```python
from build123d import *

# Parameters (mm, degrees)
F0_W     = 1.5
F0_H     = 0.7
F0_R     = 2.25
F0_H_2   = 8.6
F0_W_2   = 2.8
F1_DEPTH = 5
F2_DEPTH = 3
F3_DEPTH = 2
F4_R     = 0.74999
F5_R     = 2


# Not quite as in the source:
# - a fillet or chamfer is up to 0.001 mm smaller than in the source, because OpenCascade refuses the exact size


with BuildPart() as f1:
    # F0 (on Top) → F1 (new body)
    with BuildSketch(Plane.XY):
        Polygon((-18.8879279066, 5), (-22.8879279066, 5), (-22.8879279066, 2), (-18.8879279066, 2.46), align=None)
        Polygon((-17.3879279066, 5), (-18.8879279066, 5), (-18.8879279066, 2.46), (-17.3879279066, 2.6325), align=None)
        Polygon((-18.8879279066, 2.46), (-22.8879279066, 2), (-22.8879279066, -2), (-18.8879279066, -2.46), align=None)
        Polygon((-12.9879279066, 5), (-17.3879279066, 5), (-17.3879279066, 2.6325), (-12.9879279066, 3.1385), align=None)
        Polygon((-18.8879279066, -2.46), (-22.8879279066, -2), (-22.8879279066, -5), (-18.8879279066, -5), align=None)
        Polygon((-11.4879279066, 5), (-12.9879279066, 5), (-12.9879279066, 3.1385), (-11.4879279066, 3.311), align=None)
        Polygon((-17.3879279066, -2.6325), (-18.8879279066, -2.46), (-18.8879279066, -5), (-17.3879279066, -5), align=None)
        Polygon((-7.0879279066, 5), (-11.4879279066, 5), (-11.4879279066, 3.311), (-7.0879279066, 3.817), align=None)
        Polygon((-12.9879279066, -3.1385), (-17.3879279066, -2.6325), (-17.3879279066, -5), (-12.9879279066, -5), align=None)
        Polygon((-5.5879279066, 5), (-7.0879279066, 5), (-7.0879279066, 3.817), (-5.5879279066, 3.9895), align=None)
        Polygon((-11.4879279066, -3.311), (-12.9879279066, -3.1385), (-12.9879279066, -5), (-11.4879279066, -5), align=None)
        Polygon((-1.1879279066, 5), (-5.5879279066, 5), (-5.5879279066, 3.9895), (-2.8879279066, 4.3), (-1.1879279066, 4.3), align=None)
        Polygon((-7.0879279066, -3.817), (-11.4879279066, -3.311), (-11.4879279066, -5), (-7.0879279066, -5), align=None)
        with Locations((-0.4379279066, 4.65)):
            Rectangle(F0_W, F0_H)
        Polygon((-5.5879279066, -3.9895), (-7.0879279066, -3.817), (-7.0879279066, -5), (-5.5879279066, -5), align=None)
        Polygon((12.1120720934, 5), (0.3120720934, 5), (0.3120720934, 4.3), (3.1120720934, 4.3), (3.1120720934, -4.3), (0.3120720934, -4.3), (0.3120720934, -5), (12.1120720934, -5), align=None)
        with Locations((8.1120720934, 0)):
            Circle(F0_R, mode=Mode.SUBTRACT)
        Polygon((-2.8879279066, -4.3), (-5.5879279066, -3.9895), (-5.5879279066, -5), (-1.1879279066, -5), (-1.1879279066, -4.3), align=None)
        with Locations((-0.4379279066, -4.65)):
            Rectangle(F0_W, F0_H)
        with Locations((-0.4379279066, 0)):
            Rectangle(F0_W, F0_H_2)
        Polygon((-5.5879279066, 3.9895), (-7.0879279066, 3.817), (-7.0879279066, -3.817), (-5.5879279066, -3.9895), align=None)
        Polygon((-17.3879279066, 2.6325), (-18.8879279066, 2.46), (-18.8879279066, -2.46), (-17.3879279066, -2.6325), align=None)
        Polygon((-12.9879279066, 3.1385), (-17.3879279066, 2.6325), (-17.3879279066, -2.6325), (-12.9879279066, -3.1385), align=None)
        Polygon((-7.0879279066, 3.817), (-11.4879279066, 3.311), (-11.4879279066, -3.311), (-7.0879279066, -3.817), align=None)
        Polygon((-11.4879279066, 3.311), (-12.9879279066, 3.1385), (-12.9879279066, -3.1385), (-11.4879279066, -3.311), align=None)
        Polygon((-2.8879279066, 4.3), (-5.5879279066, 3.9895), (-5.5879279066, -3.9895), (-2.8879279066, -4.3), (-1.1879279066, -4.3), (-1.1879279066, 4.3), align=None)
        with Locations((1.7120720934, 0)):
            Rectangle(F0_W_2, F0_H_2)
    extrude(amount=-F1_DEPTH)

    # F0 (on Top) → F2 (cut)
    with BuildSketch(Plane.XY):
        Polygon((-18.8879279066, 2.46), (-22.8879279066, 2), (-22.8879279066, -2), (-18.8879279066, -2.46), align=None)
        Polygon((-17.3879279066, 2.6325), (-18.8879279066, 2.46), (-18.8879279066, -2.46), (-17.3879279066, -2.6325), align=None)
        Polygon((-12.9879279066, 3.1385), (-17.3879279066, 2.6325), (-17.3879279066, -2.6325), (-12.9879279066, -3.1385), align=None)
        Polygon((-11.4879279066, 3.311), (-12.9879279066, 3.1385), (-12.9879279066, -3.1385), (-11.4879279066, -3.311), align=None)
        Polygon((-7.0879279066, 3.817), (-11.4879279066, 3.311), (-11.4879279066, -3.311), (-7.0879279066, -3.817), align=None)
        Polygon((-5.5879279066, 3.9895), (-7.0879279066, 3.817), (-7.0879279066, -3.817), (-5.5879279066, -3.9895), align=None)
        Polygon((-2.8879279066, 4.3), (-5.5879279066, 3.9895), (-5.5879279066, -3.9895), (-2.8879279066, -4.3), (-1.1879279066, -4.3), (-1.1879279066, 4.3), align=None)
        with Locations((-0.4379279066, 0)):
            Rectangle(F0_W, F0_H_2)
        with Locations((1.7120720934, 0)):
            Rectangle(F0_W_2, F0_H_2)
    extrude(amount=-F2_DEPTH, mode=Mode.SUBTRACT)

    # F0 (on Top) → F3 (cut)
    with BuildSketch(Plane.XY):
        Polygon((-17.3879279066, 5), (-18.8879279066, 5), (-18.8879279066, 2.46), (-17.3879279066, 2.6325), align=None)
        Polygon((-11.4879279066, 5), (-12.9879279066, 5), (-12.9879279066, 3.1385), (-11.4879279066, 3.311), align=None)
        Polygon((-5.5879279066, 5), (-7.0879279066, 5), (-7.0879279066, 3.817), (-5.5879279066, 3.9895), align=None)
        with Locations((-0.4379279066, -4.65)):
            Rectangle(F0_W, F0_H)
        Polygon((-17.3879279066, -2.6325), (-18.8879279066, -2.46), (-18.8879279066, -5), (-17.3879279066, -5), align=None)
        Polygon((-11.4879279066, -3.311), (-12.9879279066, -3.1385), (-12.9879279066, -5), (-11.4879279066, -5), align=None)
        Polygon((-5.5879279066, -3.9895), (-7.0879279066, -3.817), (-7.0879279066, -5), (-5.5879279066, -5), align=None)
        with Locations((-0.4379279066, 4.65)):
            Rectangle(F0_W, F0_H)
    extrude(amount=-F3_DEPTH, mode=Mode.SUBTRACT)

    # F4 (radius 0.75 in the source; OpenCascade refuses exactly that, so slightly less here)
    f4_edges = [f1.edges().sort_by_distance(p)[0] for p in [
        (-17.387928, -3.81625, -2),
        (-11.487928, -4.1555, -2),
        (-5.587928, -4.49475, -2),
        (0.312072, -4.65, -2),
        (-18.887928, -3.73, -2),
        (-12.987928, -4.06925, -2),
        (-7.087928, -4.4085, -2),
        (-1.187928, -4.65, -2),
        (-18.887928, 3.73, -2),
        (-12.987928, 4.06925, -2),
        (-7.087928, 4.4085, -2),
        (-1.187928, 4.65, -2),
        (-17.387928, 3.81625, -2),
        (-11.487928, 4.1555, -2),
        (-5.587928, 4.49475, -2),
        (0.312072, 4.65, -2),
        (3.112072, 4.3, -1.5),
        (3.112072, -4.3, -1.5),
    ]]
    fillet(f4_edges, radius=F4_R)

    # F5
    f5_edges = [f1.edges().sort_by_distance(p)[0] for p in [
        (-22.887928, -5, -2.5),
        (-22.887928, 5, -2.5),
        (12.112072, -5, -2.5),
        (12.112072, 5, -2.5),
    ]]
    fillet(f5_edges, radius=F5_R)


solid = f1.part
```
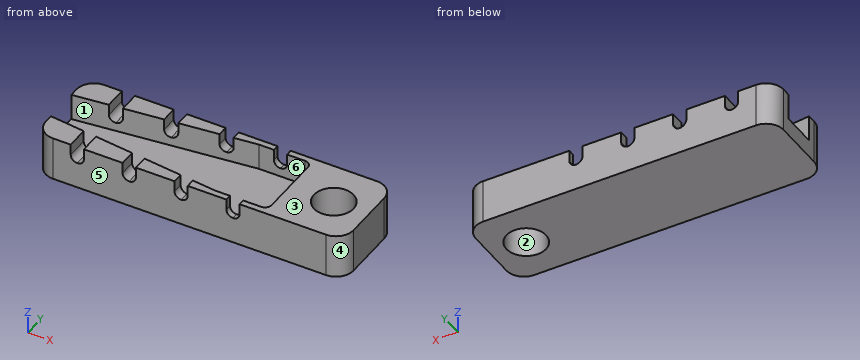
Part model, mm, in its own coordinate system. Face numbers are marked on the shaded views. A direction names the side the tool comes from. Coordinates: 2 decimals unless noted, no trailing zeros. Loops run counter-clockwise (first coordinate to the right, second up) from the corner with the lowest first, then second, coordinate; pieces in that order, holes last. Notation, with made-up numbers: (17.5, 75) - (55.5, 75) arc R13 cw to (55.5, 92) - close; hole circle Ø5 at (38.25, 23). An arc over 180 degrees is marked (long way). Write item = value, one per line. Start each with the question number.
Item 1: 3-axis set-ups, long thin cutter, end or side, ignore diameter. For the marked faces 5 and 6: which of +Z, -Z, +X, -X, +Y, -Y reach the whole face in a straight line?
Item 2: Cut at B-B, the plane y = 0. Give the cut face in (x, z), and give its area (3 significant figures).
Item 3: Cut at D-D, the plane x = 6.5. Give the cut face in (y, z), and give its area (3 significant figures).
Item 4: Cut at C-C, the plane z = -0.7. State how many separate pieces and enclosed holes the cut face has, and give its area (3 significant figures).
Item 5: Wall check: L1, parallel to X at y = -2.5, z = -0.8; L2, parallel to Y at x = 6.5, z = -1.4; L3, parallel to Z at x = -18.5, y = 0.5. Give the ranges that are in metal, low to high. Write a range as from..to.
Item 6: Flat gauge pins, fed straight in: pin 1 Ø0.8 at (y, z) = (4.5, -1) entering from +X; pin 2 Ø0.9 at (y, z) = (-0.5, -1.5) entering from -X; pin 3 Ø0.6 at (y, z) = (4.5, -1) entering from +X. Where does each tip first touch, or does it go through?
Item 7: Cut at A-A, the plane z = -3.75. Give the cut face in (x, y).
Item 8: Mould opens along Y. For the marked faces 1, 2, 3 and 4 say: released by +Y, released by -Y, zero draft, split by the parting line, or undercut.
The answers:
q1.face_5 = +Z, -Z, +X, -X, -Y
q1.face_6 = +Z
q2.outline = (-22.89, -5) - (5.86, -5) - (5.86, 0) - (3.11, 0) - (3.11, -3) - (-22.89, -3) - close; (10.36, -5) - (12.11, -5) - (12.11, 0) - (10.36, 0) - close
q2.area = 74.5 mm2
q3.outline = (-5, -5) - (-1.57, -5) - (-1.57, 0) - (-5, 0) - close; (1.57, -5) - (5, -5) - (5, 0) - (1.57, 0) - close
q3.area = 34.3 mm2
q4.separate_pieces = 9
q4.enclosed_holes = 1
q4.area = 135 mm2
q5.L1 = -22.89..-18.89, 3.11..12.11
q5.L2 = -5..-1.57, 1.57..5
q5.L3 = -5..-3
q6.pin_1 = 11.78
q6.pin_2 = 3.11
q6.pin_3 = 11.71
q7.outline = (-22.89, -3) arc R2 ccw to (-20.89, -5) - (10.11, -5) arc R2 ccw to (12.11, -3) - (12.11, 3) arc R2 ccw to (10.11, 5) - (-20.89, 5) arc R2 ccw to (-22.89, 3) - close; hole circle Ø4.5 at (8.11, 0)
q8.face_1 = undercut
q8.face_2 = undercut
q8.face_3 = zero draft
q8.face_4 = released by -Y
